from build123d import *

# Parameters (mm, degrees)
F0_W     = 52.0596802235
F0_H     = 50.2265766263
F1_DEPTH = 330
F2_DEPTH = 2000
F3_DEPTH = 2000
F4_DEPTH = 1000
F5_T     = -16


with BuildPart() as f1:
    # F0 (on Front) → F1 (new body)
    with BuildSketch(Plane.XZ):
        with Locations((26.0298401117, 25.1132883132)):
            Rectangle(F0_W, F0_H)
    extrude(amount=F1_DEPTH)

    # F2 (add): a face of the model
    f2_faces = [f1.faces().sort_by_distance(p)[0] for p in [
        (0, -165, 25.1132883132),
    ]]
    extrude(f2_faces, amount=-F2_DEPTH)

    # F3 (add): a face of the model
    f3_faces = [f1.faces().sort_by_distance(p)[0] for p in [
        (1000, -165, 0),
    ]]
    extrude(f3_faces, amount=-F3_DEPTH)

    # F4 (intersect): a face of the model
    f4_faces = [f1.faces().sort_by_distance(p)[0] for p in [
        (0, -165, 1000),
    ]]
    extrude(f4_faces, amount=-F4_DEPTH, mode=Mode.INTERSECT)

    # F5
    f5_openings = [f1.faces().sort_by_distance(p)[0] for p in [
        (500, -330, 1000),
    ]]
    offset(amount=F5_T, openings=f5_openings)


solid = f1.part
Verification items for the finished model (mm, model axes). A direction names the side the tool comes from. Round coordinates to 2 decimals unless told otherwise and drop trailing zeros. Loops run counter-clockwise (first coordinate to the right, second up) from the corner with the lowest first, then second, coordinate; pieces in that order, holes last. Notation, with made-up numbers: (48, 52) - (56, 52) arc R19 ccw to (56, 83) - close; hole circle Ø1 at (0.5, 8.25). An arc over 180 degrees is marked (long way). Use a Markdown table: item, result. Add a question column.
1. Thickness scan on probe 1 along Z at (x, y) = (658, -273); probe 2 along X at (y, z) = (-182.5, 1268); probe 3 along Y at (x, z) = (903, 1290.5). Record the ranges inside material, lowest first. Write a range as [from, to].
2. Section check C-C, the plane z = 1026. Record the boundary of the cut face in (x, y).
3. Access from +Z, -Z, +X, -X, +Y, -Y to the whole of each face (thin tool, end or side, straight path). Record for faces 1 (the face through (493, 0, 1014)), 2 (the face through (493, -171, 16)).
4. Section check A-A, the plane y = -80. Record the boundary of the cut face in (x, z).
5. Gauge pin test, flat end, axial feed: pin 1 (4 mm diameter, centred on x = 311.5, z = 342.5, fed in from -Y). Record the tip position at first contact, or that the pin passes through.
6. Section check B-B, the plane x = 433. Record the boundary of the cut face in (y, z), plus the area to 3 significant figures.
7. Release check for a two-part mould opening along Z. For faces 3 (the face through (984, -171, 986)), 4 (the face through (493, -163, 0)), 5 (the face through (493, -16, 1014)), 6 (the face through (1000, -163, 986)) record: released by +Z, released by -Z, zero draft, split by the parting line, or undercut.
Checks:
| question | item | result |
|---|---|---|
| 1 | probe 1 | z = [0, 16], [1984, 2000] |
| 1 | probe 2 | x = [0, 16], [984, 1000] |
| 1 | probe 3 | y = [-16, 0] |
| 2 | outline | (0, -330) - (16, -330) - (16, -16) - (984, -16) - (984, -330) - (1000, -330) - (1000, 0) - (0, 0) - close |
| 3 | face 1 | +Z, -Z, +X, -X, +Y |
| 3 | face 2 | -Y |
| 4 | outline | (0, 0) - (1000, 0) - (1000, 2000) - (0, 2000) - close; hole (16, 16) - (984, 16) - (984, 1984) - (16, 1984) - close |
| 5 | pin 1 | stops at y = -16 |
| 6 | outline | (-330, 0) - (0, 0) - (0, 2000) - (-330, 2000) - (-330, 1984) - (-16, 1984) - (-16, 16) - (-330, 16) - close |
| 6 | area | 42,000 mm^2 |
| 7 | face 3 | undercut |
| 7 | face 4 | released by -Z |
| 7 | face 5 | undercut |
| 7 | face 6 | zero draft |
